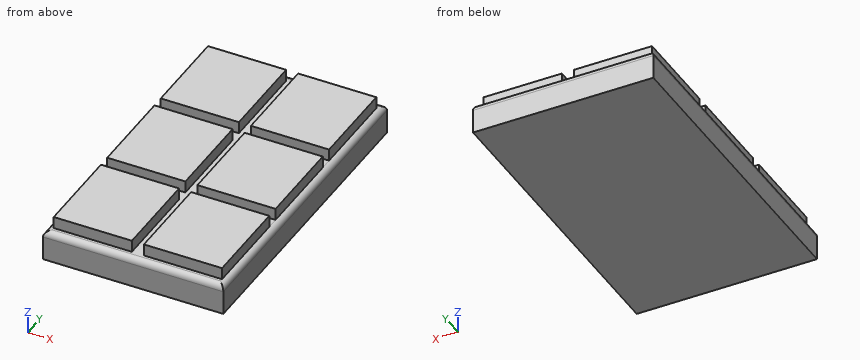
from build123d import *

# Parameters (mm, degrees)
F0_W     = 6.5
F0_H     = 15
F1_DEPTH = 7
F2_DEPTH = 5
F4_R     = 0.99999


# Not quite as in the source:
# - a fillet or chamfer is up to 0.001 mm smaller than in the source, because OpenCascade refuses the exact size
# - a feature names something its author has since deleted; it is built from what else it names


with BuildPart() as f1:
    # F0 (on Top) → F1 (new body)
    with BuildSketch(Plane.XY):
        with Locations((-4.25, 17)):
            Rectangle(F0_W, F0_H)
        with Locations((-10.75, 17)):
            Rectangle(F0_W, F0_H)
    extrude(amount=F1_DEPTH)


with BuildPart() as f1b:
    # F0 (on Top) → F1, piece 2 (new body)
    with BuildSketch(Plane.XY):
        with Locations((-10.75, 0)):
            Rectangle(F0_W, F0_H)
        with Locations((-4.25, 0)):
            Rectangle(F0_W, F0_H)
    extrude(amount=F1_DEPTH)


with BuildPart() as f1c:
    # F0 (on Top) → F1, piece 3 (new body)
    with BuildSketch(Plane.XY):
        with Locations((-4.25, -17)):
            Rectangle(F0_W, F0_H)
        with Locations((-10.75, -17)):
            Rectangle(F0_W, F0_H)
    extrude(amount=F1_DEPTH)


with BuildPart() as f1d:
    # F0 (on Top) → F1, piece 4 (new body)
    with BuildSketch(Plane.XY):
        with Locations((4.25, -17)):
            Rectangle(F0_W, F0_H)
        with Locations((10.75, -17)):
            Rectangle(F0_W, F0_H)
    extrude(amount=F1_DEPTH)


with BuildPart() as f1e:
    # F0 (on Top) → F1, piece 5 (new body)
    with BuildSketch(Plane.XY):
        with Locations((10.75, 0)):
            Rectangle(F0_W, F0_H)
        with Locations((4.25, 0)):
            Rectangle(F0_W, F0_H)
    extrude(amount=F1_DEPTH)


with BuildPart() as f1f:
    # F0 (on Top) → F1, piece 6 (new body)
    with BuildSketch(Plane.XY):
        with Locations((4.25, 17)):
            Rectangle(F0_W, F0_H)
        with Locations((10.75, 17)):
            Rectangle(F0_W, F0_H)
    extrude(amount=F1_DEPTH)


with BuildPart() as f2:
    # F0 (on Top) → F2 (new body)
    with BuildSketch(Plane.XY):
        Polygon((-7.5, 24.5), (-7.5, 26), (-15, 26), (-15, -26), (-7.5, -26), (-7.5, -24.5), (-14, -24.5), (-14, -9.5), (-7.5, -9.5), (-7.5, -7.5), (-14, -7.5), (-14, 7.5), (-7.5, 7.5), (-7.5, 9.5), (-14, 9.5), (-14, 24.5), align=None)
        Polygon((7.5, 24.5), (7.5, 26), (-7.5, 26), (-7.5, 24.5), (-1, 24.5), (-1, 9.5), (-7.5, 9.5), (-7.5, 7.5), (-1, 7.5), (-1, -7.5), (-7.5, -7.5), (-7.5, -9.5), (-1, -9.5), (-1, -24.5), (-7.5, -24.5), (-7.5, -26), (7.5, -26), (7.5, -24.5), (1, -24.5), (1, -9.5), (7.5, -9.5), (7.5, -7.5), (1, -7.5), (1, 7.5), (7.5, 7.5), (7.5, 9.5), (1, 9.5), (1, 24.5), align=None)
        Polygon((15, -26), (15, 26), (7.5, 26), (7.5, 24.5), (14, 24.5), (14, 9.5), (7.5, 9.5), (7.5, 7.5), (14, 7.5), (14, -7.5), (7.5, -7.5), (7.5, -9.5), (14, -9.5), (14, -24.5), (7.5, -24.5), (7.5, -26), align=None)
    extrude(amount=F2_DEPTH)


with BuildPart() as f1f_1:
    add(f1f.part)

    # F3: union F1b, F1c, F2, F1, F1d, F1e
    add(f1b.part)
    add(f1c.part)
    add(f2.part)
    add(f1.part)
    add(f1d.part)
    add(f1e.part)

    # F4 (radius 1 in the source; OpenCascade refuses exactly that, so slightly less here)
    f4_edges = [f1f_1.edges().sort_by_distance(p)[0] for p in [
        (-15, 0, 5),
        (0, -26, 5),
        (15, 0, 5),
        (0, 26, 5),
    ]]
    fillet(f4_edges, radius=F4_R)


solid = f1f_1.part
CAD build for the part. Positions are in the model's coordinates, mm. Round coordinates to 2 decimals unless told otherwise and drop trailing zeros. Order: outer loops, then holes, each group sorted by start corner. A loop starts at its lowest first (then second) coordinate and runs counter-clockwise, first axis right, second up. Notation, with made-up numbers: (-10.75, -39) - (45.25, -39) arc R26 cw to (45.25, -18) - close; hole circle Ø2 at (-10.75, 42.5). An arc over 180 degrees is marked (long way). Return JSON: item names as keys, results as strings.
(1) Pin check, flat tips, straight feed: pin 1 Ø0.6 at (x, z) = (8.5, 6) entering from -Y; pin 2 Ø1.6 at (y, z) = (1.5, 6) entering from +X; pin 3 Ø1.6 at (x, z) = (-4.5, 5.5) entering from -Y. Stop position of each tip, or through.
Answer key:
{"pin 1": "stops at y = -24.5", "pin 2": "stops at x = 14", "pin 3": "stops at y = -25.71"}
(2) Wall check: probe 1 along Y at (x, z) = (2.5, 6.5); probe 2 along X at (y, z) = (-7, 6.25); probe 3 along Z at (x, y) = (2.5, 8.5). Give the ranges that are in metal, low to high. Write a range as from..to.
Answer key:
{"probe 1": "y = -24.5..-9.5, -7.5..7.5, 9.5..24.5", "probe 2": "x = -14..-1, 1..14", "probe 3": "z = 0..5"}
(3) Cut at D-D (y = 9). Give the cut face in (x, z).
Answer key:
{"outline": "(-15, 0) - (15, 0) - (15, 4) arc R1 ccw to (14, 5) - (-14, 5) arc R1 ccw to (-15, 4) - close"}
(4) Cut at C-C (x = -12). Give the cut face in (y, z).
Answer key:
{"outline": "(-26, 0) - (26, 0) - (26, 4) arc R1 ccw to (25, 5) - (24.5, 5) - (24.5, 7) - (9.5, 7) - (9.5, 5) - (7.5, 5) - (7.5, 7) - (-7.5, 7) - (-7.5, 5) - (-9.5, 5) - (-9.5, 7) - (-24.5, 7) - (-24.5, 5) - (-25, 5) arc R1 ccw to (-26, 4) - close"}
(5) Cut at A-A (z = 5.75). Give the cut face in (x, y), then the cut area to 3 significant figures.
Answer key:
{"outline": "(-14, -24.5) - (-1, -24.5) - (-1, -9.5) - (-14, -9.5) - close; (-14, -7.5) - (-1, -7.5) - (-1, 7.5) - (-14, 7.5) - close; (-14, 9.5) - (-1, 9.5) - (-1, 24.5) - (-14, 24.5) - close; (1, -24.5) - (14, -24.5) - (14, -9.5) - (1, -9.5) - close; (1, -7.5) - (14, -7.5) - (14, 7.5) - (1, 7.5) - close; (1, 9.5) - (14, 9.5) - (14, 24.5) - (1, 24.5) - close", "area": "1,170 mm^2"}
